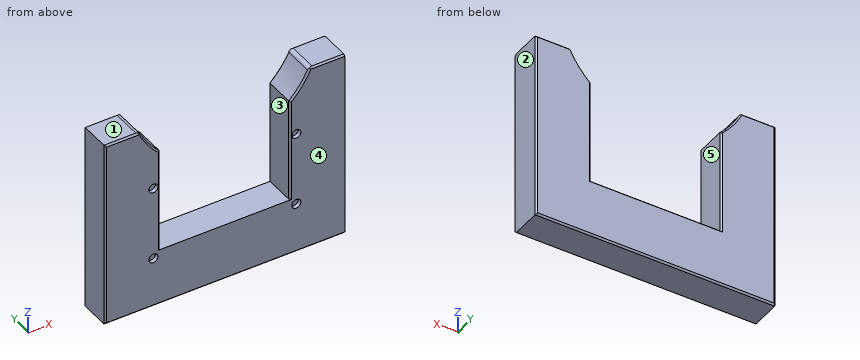
Autodesk Inventor part; units mm, degrees
ref_plane "YZ Plane" through (0, 0, 0) normal (1, 0, 0) x (0, 1, 0)
ref_plane "XZ Plane" through (0, 0, 0) normal (0, 1, 0) x (-1, 0, 0)
ref_plane "XY Plane" through (0, 0, 0) normal (0, 0, 1) x (1, 0, 0)
sketch "Sketch1" plane through (0, 0, 0) normal (0, 1, 0) x (-1, 0, 0)
  line L0 (73, 70) -> (-73, 70)
  line L1 (-73, 70) -> (-73, -70)
  line L2 (-73, -70) -> (73, -70)
  line L3 (73, -70) -> (73, 70)
  line L4 (73, 70) -> (-73, -70) construction
  line L5 (-73, 70) -> (73, -70) construction
  line L6 (-73, -70) -> (73, -70)
  line L7 (73, -70) -> (73, 45)
  line L8 (73, 45) -> (-73, 45)
  line L9 (-73, 45) -> (-73, -70)
  circle A0 centre (0, 70) radius 57.5
  line L10 (39.5, 175) -> (-39.5, 175)
  line L11 (-39.5, 175) -> (-39.5, -35)
  line L12 (-39.5, -35) -> (39.5, -35)
  line L13 (39.5, -35) -> (39.5, 175)
  line L14 (39.5, 175) -> (-39.5, -35) construction
  line L15 (-39.5, 175) -> (39.5, -35) construction
  point P0 (0, 0)
  point P1 (-39.5, 28.2148)
  point P2 (-51.7808, 45)
  point P3 (51.7808, 45)
  point P4 (39.5, 28.2148)
  dimension "d0" = 146
  dimension "d1" = 140
  dimension "d2" = 115
  dimension "d3" = 115
  dimension "d4" = 210
  dimension "d5" = 79
extrude "Extrusion1" add sketch "Sketch1" along normal blind 20 contours L3 L2 L1 L8 A0 L11 L12 L13
sketch "Sketch2" plane through (0, 0, 0) normal (0, -1, 0) x (1, 0, 0)
  circle A0 centre (-43.5, -39) radius 2.75
  circle A1 centre (43.5, -39) radius 2.75
  line L0 (-39.5, 28.2148) -> (-39.5, -35)
  line L1 (-39.5, -35) -> (39.5, -35)
  line L2 (39.5, -35) -> (39.5, 28.2148)
  circle A2 centre (43.5, 6) radius 2.75
  circle A3 centre (-43.5, 6) radius 2.75
  point P0 (0, 0)
  dimension "d8" = 5.5
  dimension "d9" = 5.5
  dimension "d10" = 4
  dimension "d11" = 4
  dimension "d12" = 4
  dimension "d13" = 4
  dimension "d14" = 5.5
  dimension "d15" = 5.5
  dimension "d16" = 45
  dimension "d17" = 45
extrude "Extrusion2" cut sketch "Sketch2" against normal blind 2.5
chamfer "Chamfer1" distance 1 angle 45 18 edges at (-46.4056, 0, 36.0475) (-46.4056, 20, 36.0475) (-62.3904, 20, 45) (-62.3904, 0, 45) (46.4056, 0, 36.0475) (46.4056, 20, 36.0475) (62.3904, 20, 45) (62.3904, 0, 45) (73, 20, -12.5) (-73, 20, -12.5) (-73, 0, -12.5) (0, 20, -70) (0, 0, -70) (-39.5, 20, -3.3926) (-39.5, 0, -3.3926) (0, 20, -35) (39.5, 20, -3.3926) (39.5, 0, -3.3926)
fillet "Fillet1" radius 3 2 edges at (51.7808, 10, 45) (-51.7808, 10, 45)
properties part number "Spacer 1"
Check sheet for the modelled part. Datum: model origin and axes. Units: mm. Face numbers are marked on the shaded views. A direction names the side the tool comes from. Coordinates: 2 decimals unless noted, no trailing zeros. Write each loop counter-clockwise with the first axis right and the second up, starting at its lowest first coordinate (ties: lowest second). Pieces come first, ordered by that corner, then holes. Notation, with made-up numbers: M -7,78.25 L 48,78.25 A28 cw 48,104.25 Z; hole C 38.5,-10 d9. An arc over 180 degrees is marked long. Answer as CSV lines item,"result".
Q1. Cross-section at D-D (z = 26). Record the boundary of the cut face in (x, y).
Check result:
outline,"M -73,1 L -72,0 L -40.5,0 L -39.5,1 L -39.5,19 L -40.5,20 L -72,20 L -73,19 Z; M 39.5,1 L 40.5,0 L 73,0 L 73,19 L 72,20 L 40.5,20 L 39.5,19 Z"
Q2. Go/stop test with flat-tipped pins: pin 1 (4 mm diameter, centred on x = 7.5, y = 11.5, fed in from +Z); pin 2 (3.5 mm diameter, centred on x = 43.5, z = 6, fed in from -Y); pin 3 (10 mm diameter, centred on x = -46.5, y = 16.5, fed in from +Z). Record where each tip stops, or that it passes through.
Check result:
pin 1,"z = -35"
pin 2,"y = 2.5"
pin 3,"z = 44.11"
Q3. Mould release check, pull along X, two halves, no side actions. Record for the marked faces 1, 2 and 3: released by +X, released by -X, zero draft, split by the parting line, or undercut.
Check result:
face 1,"zero draft"
face 2,"released by +X"
face 3,"undercut"
Q4. Cross-section at B-B (y = 14.75). Record the boundary of the cut face in (x, z).
Check result:
outline,"M -73,-70 L 73,-70 L 73,45 L 53.63,45 A3 ccw 50.97,43.39 A57.5 cw 39.5,28.21 L 39.5,-35 L -39.5,-35 L -39.5,28.21 A57.5 cw -50.97,43.39 A3 ccw -53.63,45 L -73,45 Z"
Q5. Set-up check for the marked faces 4 and 5: record each of +Z, -Z, +X, -X, +Y, -Y from which the full face is reachable in a straight line by a thin tool's end or side.
Check result:
face 4,"+Z, -Z, +X, -X, -Y"
face 5,"+Z, +Y, -Y"
Q6. Cross-section at A-A (z = 6). Record the boundary of the cut face in (x, y).
Check result:
outline,"M -73,1 L -72,0 L -46.25,0 L -46.25,2.5 L -40.75,2.5 L -40.75,0 L -40.5,0 L -39.5,1 L -39.5,19 L -40.5,20 L -72,20 L -73,19 Z; M 39.5,1 L 40.5,0 L 40.75,0 L 40.75,2.5 L 46.25,2.5 L 46.25,0 L 73,0 L 73,19 L 72,20 L 40.5,20 L 39.5,19 Z"
Q7. Material ranges on probe 1 along Z at (x, y) = (43.5, 1.7); probe 2 along X at (y, z) = (14.5, 23.5); probe 3 along Z at (x, y) = (43.5, 0.6), recorded low to high. Write a range as from..to.
Check result:
probe 1,"-70..-41.75, -36.25..3.25, 8.75..32.4"
probe 2,"-73..-39.5, 39.5..73"
probe 3,"-69.6..-41.75, -36.25..3.25, 8.75..31.79"
Q8. Cross-section at C-C (x = -10). Record the boundary of the cut face in (y, z), then the cut area to 4 significant figures.
Check result:
outline,"M 0,-69 L 1,-70 L 19,-70 L 20,-69 L 20,-36 L 19,-35 L 0,-35 Z"
area,"698.5 mm^2"
